Model file for the job. Use its own axes, mm. Round coordinates to 2 decimals unless told otherwise and drop trailing zeros. Write item = value, one per line.
```python
from build123d import *

# Parameters (mm, degrees)
BOSS_EXTRUDE1_DEPTH = 30
SKETCH2_R           = 55
BOSS_EXTRUDE2_DEPTH = 5
SKETCH3_R           = 30
BOSS_EXTRUDE3_DEPTH = 10
SKETCH4_R           = 5
CUT_EXTRUDE4_DEPTH  = 20
SKETCH5_R           = 3
CUT_EXTRUDE5_DEPTH  = 33.082590237
FILLET1_R           = 2.5
FILLET2_R           = 1.5
DOME1_FACE_RADIUS   = 27.5
DOME1_HEIGHT        = 4


with BuildPart() as part:
    # Sketch1 → Boss-Extrude1 (new body)
    with BuildSketch(Plane(origin=(-0.609266147, 0, 59.996906543), x_dir=(0.99993435, 0.005309042, 0.010154293), z_dir=(-0.010154436, 0, 0.999948442))):
        with BuildLine():
            Line((13.092334874, 339.479342253), (-71.283345055, 360.871198017))
            ThreePointArc((-71.283345055, 360.871198017), (-156.616646458, 294.835639545), (-71.989316722, 227.897740169))
            Line((-71.989316722, 227.897740169), (12.608744127, 248.392494546))
            ThreePointArc((12.608744127, 248.392494546), (48.482712148, 293.74674302), (13.092334874, 339.479342253))
        make_face()
    extrude(amount=BOSS_EXTRUDE1_DEPTH)

    # Sketch2 → Boss-Extrude2 (add)
    with BuildSketch(Plane(origin=(-0.91389922, 0, 89.995359815), x_dir=(0.99993435, 0.005309042, 0.010154293), z_dir=(-0.010154436, 0, 0.999948442))):
        with Locations((-88.433233056, 294.473645815)):
            Circle(SKETCH2_R)
    extrude(amount=BOSS_EXTRUDE2_DEPTH)

    # Sketch3 → Boss-Extrude3 (add)
    with BuildSketch(Plane(origin=(-0.964671399, 0, 94.995102027), x_dir=(0.99993435, 0.005309042, 0.010154293), z_dir=(-0.010154436, 0, 0.999948442))):
        with Locations((-88.433233056, 294.473645815)):
            Circle(SKETCH3_R)
    extrude(amount=BOSS_EXTRUDE3_DEPTH)

    # Sketch4 → Cut-Extrude4 (cut)
    with BuildSketch(Plane(origin=(-0.91389922, 0, 89.995359815), x_dir=(0.99993435, 0.005309042, 0.010154293), z_dir=(-0.010154436, 0, 0.999948442))):
        with Locations((-1.318283572, 329.011635606)):
            Circle(SKETCH4_R)
        with Locations((1.375398384, 259.063482824)):
            Circle(SKETCH4_R)
    extrude(amount=-CUT_EXTRUDE4_DEPTH, mode=Mode.SUBTRACT)

    # Sketch5 → Cut-Extrude5 (cut, through all)
    with BuildSketch(Plane(origin=(-0.91389922, 0, 89.995359815), x_dir=(0.99993435, 0.005309042, 0.010154293), z_dir=(-0.010154436, 0, 0.999948442))):
        with Locations((-1.318283572, 329.011635606)):
            Circle(SKETCH5_R)
        with Locations((1.375398384, 259.063482824)):
            Circle(SKETCH5_R)
    extrude(amount=-CUT_EXTRUDE5_DEPTH, mode=Mode.SUBTRACT)

    # Fillet1
    fillet1_edges = [part.edges().sort_by_distance(p)[0] for p in [
        (-159.085477995, 294, 88.389133863),
        (-145.951780521, 293.708002671, 93.522763829),
        (-31.866493678, 237.984134176, 89.681037477),
        (-121.054966127, 293.84072873, 103.776105569),
        (46.006196549, 294, 90.47183148),
        (-31.866493678, 350.015865824, 89.681037477),
    ]]
    fillet(fillet1_edges, radius=FILLET1_R)

    # Fillet2
    fillet2_edges = [part.edges().sort_by_distance(p)[0] for p in [
        (-8.978414644, 328.973454788, 89.913464989),
        (-5.91357097, 259.040588662, 89.944588352),
    ]]
    fillet(fillet2_edges, radius=FILLET2_R)

    # Dome1: a dome of height H over a round flat face of radius A is a cap of a sphere of radius (A * A + H * H) / (2 * H)
    dome1_r = (DOME1_FACE_RADIUS * DOME1_FACE_RADIUS + DOME1_HEIGHT * DOME1_HEIGHT) / (2 * DOME1_HEIGHT)
    dome1_base = Plane((-91.056935626, 294, 104.080734349), z_dir=(0.010154436, 0, -0.999948442))
    with Locations(dome1_base.offset(DOME1_HEIGHT - dome1_r)):
        dome1_ball = Sphere(dome1_r, mode=Mode.PRIVATE)
    add(split(dome1_ball, bisect_by=dome1_base, keep=Keep.TOP, mode=Mode.PRIVATE), mode=Mode.SUBTRACT)


solid = part.part
```
1) Mould opens along X. For faces 1 (the face through (46.165, 293.128, 74.03)), 2 (the face through (-4.36, 326.068, 65.029)), 3 (the face through (-158.896, 295.739, 71.948)) say: +X half, -X half, draft (parallel to the pull), parting line (faces both ways), or undercut.
Conclusion:
face_1 = +X half
face_2 = undercut
face_3 = parting line
2) Cut at A-A (z = 74.5). Give the number of separate pieces and of enclosed holes in the cut face, and give its area (3 significant figures).
Conclusion:
separate_pieces = 1
enclosed_holes = 2
area = 21,300 mm^2
3) Wall check: line 1 along X through (y, z) = (259, 65); line 2 along Y through (x, z) = (-8.5, 86.5); line 3 along Y through (x, z) = (2.5, 89). Give the ranges that are in metal, low to high.
Conclusion:
line_1 = -149.23 to -3.66, 2.34 to 30.59
line_2 = 243.77 to 326.94, 331.06 to 344.23
line_3 = 246.99 to 255.3, 262.83 to 341.01
4) Flat gauge pins, fed straight in: pin 1 Ø10 at (y, z) = (253.5, 64.5) entering from +X; pin 2 Ø10 at (y, z) = (271.5, 71.5) entering from +X; pin 3 Ø8 at (y, z) = (310.5, 85) entering from -X. Where does each tip first touch, or does it go through?
Conclusion:
pin_1 = 30.03
pin_2 = 42.81
pin_3 = -157.9
